Work out the finished part from the listing and answer in its coordinate system (mm). Round coordinates to 2 decimals unless told otherwise and drop trailing zeros. Order: outer loops, then holes, each group sorted by start corner. A loop starts at its lowest first (then second) coordinate and runs counter-clockwise, first axis right, second up. Notation, with made-up numbers: (-35, -1) -> (-13, -1) arc R19 ccw to (-13, 29) -> close; hole circle Ø3 at (69.5, -14.75). An arc over 180 degrees is marked (long way). Use a Markdown table: item, result. Add a question column.
Item 1: A flat-ended cylindrical pin translates along its axis: P1, Ø3, axis at x = 12.7, y = 88.9, coming from the -Z side. Find the tip coordinate at first contact, or state that the pin passes through.
Item 2: Find the intervals of material crossed by L1, parallel to X at y = 12.7, z = 3; L2, parallel to X at y = 50.8, z = 3.5; L3, parallel to Y at x = 12.7, z = 4.5, in increasing order. Write a range as [from, to].
Item 3: A cutting plane is placed at A-A, the plane y = 50.8. Determine the outline of the cut face in (x, z), plus the area to 3 significant figures.
Autodesk Inventor part; units mm, degrees
ref_plane "YZ Plane" through (0, 0, 0) normal (1, 0, 0) x (0, 1, 0)
ref_plane "XZ Plane" through (0, 0, 0) normal (0, 1, 0) x (-1, 0, 0)
ref_plane "XY Plane" through (0, 0, 0) normal (0, 0, 1) x (1, 0, 0)
sketch "Sketch1" plane through (0, 0, 0) normal (0, 0, 1) x (1, 0, 0)
  line L0 (12.7, 0) -> (266.7, 0)
  line L1 (279.4, 12.7) -> (279.4, 88.9)
  line L2 (266.7, 101.6) -> (12.7, 101.6)
  line L3 (0, 88.9) -> (0, 12.7)
  arc A0 (3.175, 101.6) -> (0, 98.425) centre (3.175, 98.425) ccw
  arc A1 (266.7, 0) -> (279.4, 12.7) centre (266.7, 12.7) ccw
  arc A2 (12.7, 101.6) -> (0, 88.9) centre (12.7, 88.9) ccw
  arc A3 (0, 12.7) -> (12.7, 0) centre (12.7, 12.7) ccw
  arc A4 (279.4, 88.9) -> (266.7, 101.6) centre (266.7, 88.9) ccw
  point P0 (0, 0)
  point P1 (279.4, 101.6)
  point P2 (279.4, 0)
  point P3 (0, 101.6)
  dimension "d0" = 279.4
  dimension "d1" = 101.6
  dimension "d2" = 3.175
  dimension "d3" = 12.7
  dimension "d28" = 12.7
extrude "Extrusion1" add sketch "Sketch1" along normal blind 12.7
sketch "Sketch2" plane through (0, 0, 12.7) normal (0, 0, 1) x (1, 0, 0)
  point P0 (0, 0)
sketch "Sketch3" plane through (0, 0, 12.7) normal (0, 0, 1) x (1, 0, 0)
  line L0 (0, 88.9) -> (0, 12.7)
  line L1 (279.4, 12.7) -> (279.4, 88.9)
  line L2 (266.7, 101.6) -> (12.7, 101.6)
  point P0 (0, 0)
  point P1 (11.0744, 50.8)
  point P2 (38.1, 50.8)
  point P3 (268.2748, 50.8)
  point P4 (139.7, 50.8)
  point P5 (279.4, 101.6)
  dimension "d6" = 11.0744
  dimension "d7" = 38.1
  dimension "d8" = 139.7
  dimension "d9" = 11.1252
  dimension "d10" = 50.8
  dimension "d11" = 50.8
  dimension "d12" = 50.8
  dimension "d13" = 50.8
hole "Hole1" at (11.0744, 50.8, 12.7) at (268.2748, 50.8, 12.7) direction (0, 0, -1) diameter 6.35 end through all countersink diameter 12.7 countersink angle 82
hole "Hole2" at (38.1, 50.8, 12.7) at (139.7, 50.8, 12.7) direction (0, 0, -1) diameter 7.9375 end through all
sketch "Sketch4" plane through (0, 0, 12.7) normal (0, 0, 1) x (1, 0, 0)
  point P0 (0, 0)
sketch "Sketch5" plane through (0, 0, 0) normal (0, 0, -1) x (-1, 0, 0)
  point P0 (0, 0)
hole "Hole3" at (266.7, 88.9, 0) at (266.7, 12.7, 0) at (12.7, 12.7, 0) at (12.7, 88.9, 0) direction (0, 0, 1) diameter 3.302 end through all
properties part number "AW5.5aBasePlate"
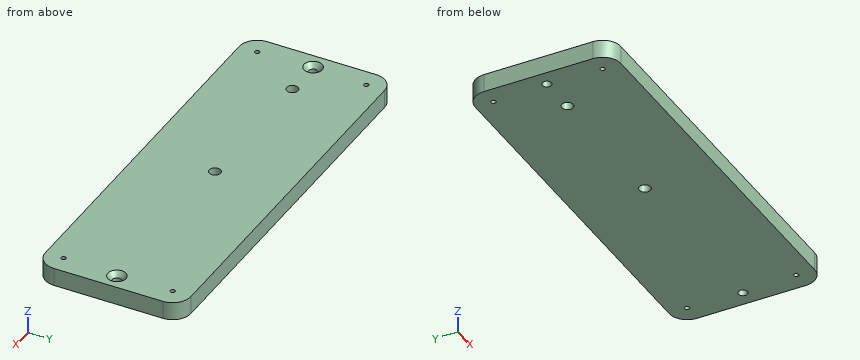
Reported:
| question | item | result |
|---|---|---|
| 1 | P1 | through |
| 2 | L1 | [0, 11.05], [14.35, 265.05], [268.35, 279.4] |
| 2 | L2 | [0, 7.9], [14.25, 34.13], [42.07, 135.73], [143.67, 265.1], [271.45, 279.4] |
| 2 | L3 | [0, 11.05], [14.35, 48.07], [53.53, 87.25], [90.55, 101.6] |
| 3 | outline | (0, 0) -> (7.9, 0) -> (7.9, 9.05) -> (4.72, 12.7) -> (0, 12.7) -> close; (14.25, 0) -> (34.13, 0) -> (34.13, 12.7) -> (17.42, 12.7) -> (14.25, 9.05) -> close; (42.07, 0) -> (135.73, 0) -> (135.73, 12.7) -> (42.07, 12.7) -> close; (143.67, 0) -> (265.1, 0) -> (265.1, 9.05) -> (261.92, 12.7) -> (143.67, 12.7) -> close; (271.45, 0) -> (279.4, 0) -> (279.4, 12.7) -> (274.62, 12.7) -> (271.45, 9.05) -> close |
| 3 | area | 3,160 mm² |
